Design review of the part shown in the three views and the two pictorial views. Dimensions are in mm from the part's minimum x, y and z. Round coordinates to 2 decimals unless told otherwise and drop trailing zeros. Loops run counter-clockwise (first coordinate to the right, second up) from the corner with the lowest first, then second, coordinate; pieces in that order, holes last. Notation, with made-up numbers: (-19, 48) -> (-12, 48) arc R17 ccw to (-12, 78) -> close; hole circle Ø8 at (14.25, 61). An arc over 180 degrees is marked (long way). Write each question's results on one line, items separated by ' | '. Start each with the question number.
Item 1: We need section A-A (x = 88). Give the boundary of the cut face in (y, z).
Item 2: We need section C-C (y = 1). Give the number of separate pieces and of enclosed holes in the cut face, and give its area (3 significant figures).
Item 3: We need section B-B (z = 27). Give the boundary of the cut face in (x, y).
Item 4: Clearance check with flat-ended pins moving along their axes: pin 1 Ø2 at (x, y) = (2.5, 2) entering from -Z; pin 2 Ø2 at (x, z) = (185, 20) entering from -Y; pin 3 Ø2 at (y, z) = (1, 133) entering from -X; pin 4 Ø2 at (y, z) = (1.5, 90) entering from +X. State where each tip first meets the part, or that it passes through.
Item 5: For L1, parallel to X at y = 2, z = 116; L2, parallel to X at y = 2.15, z = 20; L3, parallel to Z at x = 185, y = 2.3, list the stretches that pass through material, from the lowest coordinate up. Write a range as from..to.
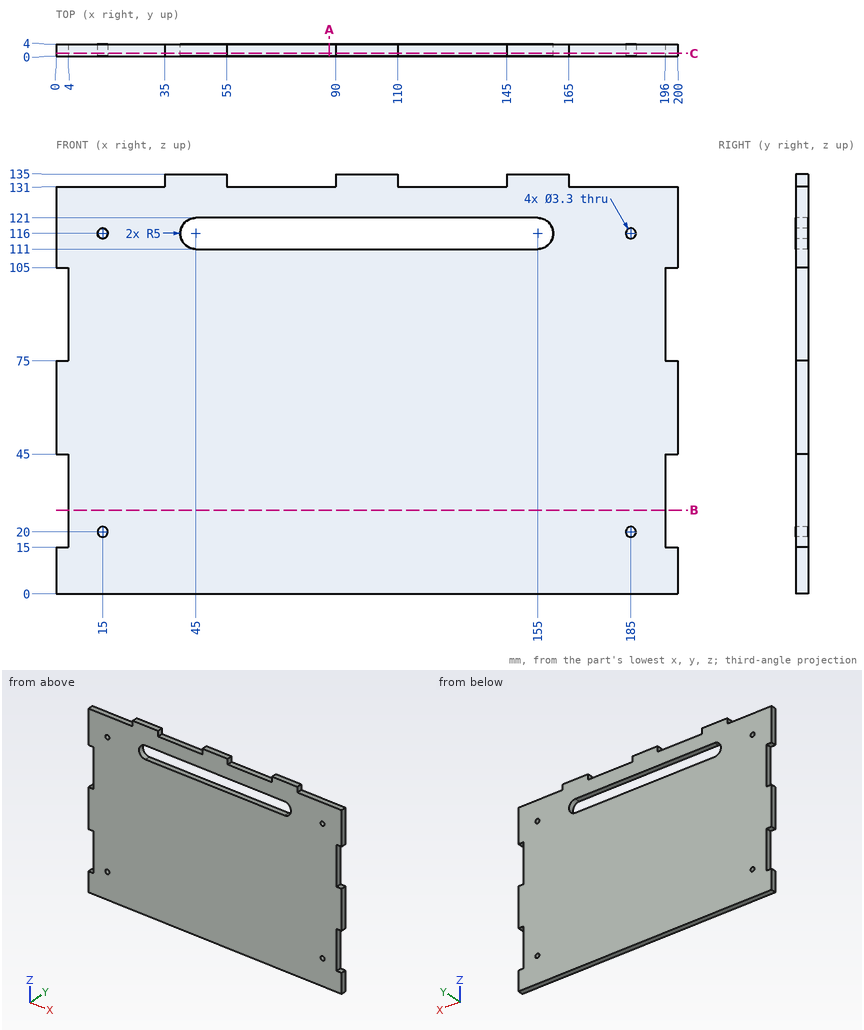
Here are the results:
1) outline: (0, 0) -> (4, 0) -> (4, 111) -> (0, 111) -> close; (0, 121) -> (4, 121) -> (4, 131) -> (0, 131) -> close
2) separate pieces: 1 | enclosed holes: 5 | area: 24,700 mm2
3) outline: (4, 0) -> (196, 0) -> (196, 4) -> (4, 4) -> close
4) pin 1: stops at z = 0 | pin 2: passes through | pin 3: stops at x = 35 | pin 4: stops at x = 196
5) L1: x = 0..13.35, 16.65..40, 160..183.35, 186.65..200 | L2: x = 4..13.35, 16.65..183.35, 186.65..196 | L3: z = 0..18.35, 21.65..114.35, 117.65..131
